from build123d import *

# Parameters (mm, degrees)
F0_W      = 60
F0_H      = 60
F1_DEPTH  = 60
F2_R      = 3
F4_DEPTH  = 5
F5_R      = 22.5
F6_DEPTH  = 5
F7_R      = 22.5
F8_DEPTH  = 4
F9_R      = 22.5
F10_DEPTH = 5
F11_R     = 22.5
F12_DEPTH = 5
F13_R     = 22.5
F14_DEPTH = 5


with BuildPart() as f1:
    # F0 (on Top) → F1 (new body)
    with BuildSketch(Plane.XY):
        with Locations((30, 30)):
            Rectangle(F0_W, F0_H)
    extrude(amount=F1_DEPTH)

    # F2
    f2_edges = [f1.edges().sort_by_distance(p)[0] for p in [
        (0, 30, 60),
        (30, 0, 60),
        (60, 30, 60),
        (30, 60, 60),
        (0, 60, 30),
        (0, 0, 30),
        (0, 30, 0),
        (60, 60, 30),
        (30, 60, 0),
        (60, 0, 30),
        (60, 30, 0),
        (30, 0, 0),
    ]]
    fillet(f2_edges, radius=F2_R)

    # F3 (on face) → F4 (cut)
    with BuildSketch(Plane.XY.offset(60)):
        with BuildLine():
            ThreePointArc((52.5, 30), (38.6103772282, 50.7872894815), (14.0900974233, 45.9099025767))
            Line((14.0900974233, 45.9099025767), (45.9099025767, 14.0900974233))
            ThreePointArc((45.9099025767, 14.0900974233), (50.7872894815, 21.3896227718), (52.5, 30))
        make_face()
        with BuildLine():
            Line((45.9099025767, 14.0900974233), (14.0900974233, 45.9099025767))
            ThreePointArc((14.0900974233, 45.9099025767), (14.0900974233, 14.0900974233), (45.9099025767, 14.0900974233))
        make_face()
    extrude(amount=-F4_DEPTH, mode=Mode.SUBTRACT)

    # F5 (on face) → F6 (cut)
    with BuildSketch(Plane.YZ.offset(60)):
        with Locations((30, 30)):
            Circle(F5_R)
    extrude(amount=-F6_DEPTH, mode=Mode.SUBTRACT)

    # F7 (on face) → F8 (join)
    with BuildSketch(Plane.XZ):
        with Locations((30, 30)):
            Circle(F7_R)
    extrude(amount=F8_DEPTH)

    # F9 (on face) → F10 (cut)
    with BuildSketch(Plane(origin=(0, 60, 0), x_dir=(-1, 0, 0), z_dir=(0, 1, 0))):
        with Locations((-30, 30)):
            Circle(F9_R)
    extrude(amount=-F10_DEPTH, mode=Mode.SUBTRACT)

    # F11 (on face) → F12 (cut)
    with BuildSketch(Plane(origin=(0, 0, 0), x_dir=(0, -1, 0), z_dir=(-1, 0, 0))):
        with Locations((-30, 30)):
            Circle(F11_R)
    extrude(amount=-F12_DEPTH, mode=Mode.SUBTRACT)

    # F13 (on face) → F14 (cut)
    with BuildSketch(Plane(origin=(0, 0, 0), x_dir=(1, 0, 0), z_dir=(0, 0, -1))):
        with Locations((30, -30)):
            Circle(F13_R)
    extrude(amount=-F14_DEPTH, mode=Mode.SUBTRACT)


solid = f1.part
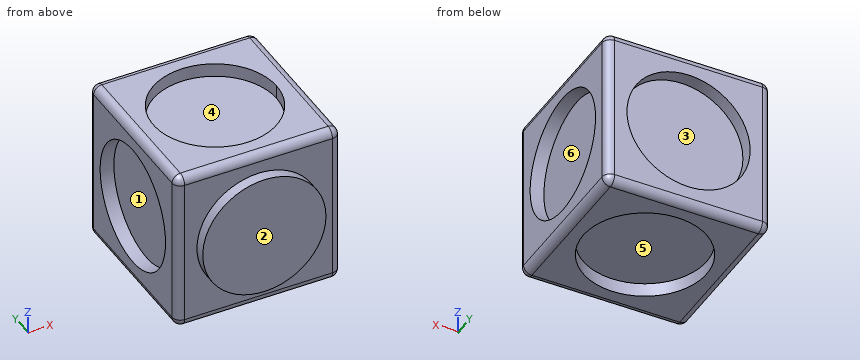
Source: CAD feature listing. Evaluate the final solid. Frame: model axes, mm. Face numbers are marked on the shaded views. A direction names the side the tool comes from. Give positions to 0.01 mm unless a question says otherwise; leave off trailing zeros. Loops run counter-clockwise (first coordinate to the right, second up) from the corner with the lowest first, then second, coordinate; pieces in that order, holes last. Notation, with made-up numbers: (6.5, 10) -> (32.5, 10) arc R11 ccw to (32.5, 30) -> close; hole circle Ø2 at (23, -20). An arc over 180 degrees is marked (long way). Use a Markdown table: item, result. Add a question column.
1) Section query A-A, the plane x = 30. Return the cut outline in (y, z), then the cut area to 3 significant figures.
2) Reachability of the marked faces 4, 5 and 6 from +Z, -Z, +X, -X, +Y, -Y: full face, straight path, thin tool, end or side. Return the list, or none.
3) Pull-direction query (Y, two-part tool) for the marked faces 1, 2 and 3; classes: +Y half, -Y half, draft (parallel to the pull), parting line (faces both ways), or undercut.
4) First-contact query: pin 1 (1.5 mm diameter, centred on y = 43.5, z = 39.5, fed in from -X); pin 2 (10 mm diameter, centred on y = 15, z = 45.5, fed in from +X); pin 3 (13.5 mm diameter, centred on y = 36.5, z = 29, fed in from +X); pin 4 (8 mm diameter, centred on x = 38, z = 33, fed in from +Y). Flat tips, straight axial feed; report the tip coordinate or a pass-through.
5) Section query B-B, the plane z = 30. Return the cut outline in (x, y), then the cut area to 3 significant figures.
6) Line query: line 1 along Z through (x, y) = (56.2, 30); line 2 along X through (y, z) = (34, 33); line 3 along Y through (x, z) = (15, 34). Output: solid intervals per line, ascending. Write a range as [from, to].
Numbers:
| question | item | result |
|---|---|---|
| 1 | outline | (-4, 7.5) -> (0, 7.5) -> (0, 3) arc R3 ccw to (3, 0) -> (7.5, 0) -> (7.5, 5) -> (52.5, 5) -> (52.5, 0) -> (57, 0) arc R3 ccw to (60, 3) -> (60, 7.5) -> (55, 7.5) -> (55, 52.5) -> (60, 52.5) -> (60, 57) arc R3 ccw to (57, 60) -> (52.5, 60) -> (52.5, 55) -> (7.5, 55) -> (7.5, 60) -> (3, 60) arc R3 ccw to (0, 57) -> (0, 52.5) -> (-4, 52.5) -> close |
| 1 | area | 3,100 mm2 |
| 2 | face 4 | +Z |
| 2 | face 5 | -Z |
| 2 | face 6 | +X |
| 3 | face 1 | undercut |
| 3 | face 2 | -Y half |
| 3 | face 3 | +Y half |
| 4 | pin 1 | stops at x = 5 |
| 4 | pin 2 | stops at x = 60 |
| 4 | pin 3 | stops at x = 55 |
| 4 | pin 4 | stops at y = 55 |
| 5 | outline | (0, 3) arc R3 ccw to (3, 0) -> (7.5, 0) -> (7.5, -4) -> (52.5, -4) -> (52.5, 0) -> (57, 0) arc R3 ccw to (60, 3) -> (60, 7.5) -> (55, 7.5) -> (55, 52.5) -> (60, 52.5) -> (60, 57) arc R3 ccw to (57, 60) -> (52.5, 60) -> (52.5, 55) -> (7.5, 55) -> (7.5, 60) -> (3, 60) arc R3 ccw to (0, 57) -> (0, 52.5) -> (5, 52.5) -> (5, 7.5) -> (0, 7.5) -> close |
| 5 | area | 3,100 mm2 |
| 6 | line 1 | z = [0, 7.5], [52.5, 60] |
| 6 | line 2 | x = [5, 55] |
| 6 | line 3 | y = [-4, 55] |
